Geometry: final body of the model. Coordinates: model frame, mm. Face numbers are marked on the shaded views. A direction names the side the tool comes from. Give positions to 0.01 mm unless a question says otherwise; leave off trailing zeros. Write each loop counter-clockwise with the first axis right and the second up, starting at its lowest first coordinate (ties: lowest second). Pieces come first, ordered by that corner, then holes.
Q1. Section A-A (y = 0). Return the cut outline in (x, z).
Q2. Mould query, pull axis Y, two halves, no side actions, for the marked faces 3, 4 and 5. Classes: +Y half, -Y half, draft (parallel to the pull), parting line (faces both ways), or undercut.
Q3. Section B-B (x = -35). Return the cut outline in (y, z).
Q4. Pin query (flat end, axial travel): pin 1 Ø5 at (y, z) = (-19, 38.5) entering from +X; pin 2 Ø1.4 at (x, y) = (0.5, -45.5) entering from -Z; pin 3 Ø6 at (x, y) = (-18.5, -7.5) entering from +Z; pin 4 Ø4 at (x, z) = (3, 8) entering from -Y. Return the tip coordinate at first contact, or that it passes through.
Q5. Section C-C (z = 40). Return the cut outline in (x, y).
Q6. Line query: line 1 (Y direction, x = 0, z = 55.5); line 2 (Z direction, x = 30, y = -27); line 3 (Y direction, x = 5, z = 57.5). Output: solid intervals per line, ascending.
Q7. Reachability of the marked faces 1 and 2 from +Z, -Z, +X, -X, +Y, -Y: full face, straight path, thin tool, end or side. Return the list, or none.
Q8. Section D-D (y = -37). Return the cut outline in (x, z).
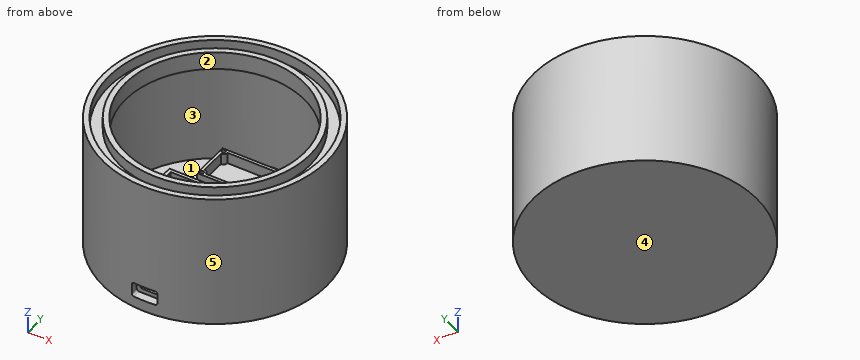
Autodesk Fusion 360 part; units mm, degrees
sketch "Boceto1" plane through (0, 0, 0) normal (0, 0, 1) x (1, 0, 0)
  circle A0 centre (0, 0) radius 50
  dimension "d4" = 100
extrude "Extruir1" add sketch "Boceto1" along normal blind 60
sketch "Boceto2" plane through (0, 0, 60) normal (0, 0, 1) x (-1, 0, 0)
  circle A0 centre (0, 0) radius 50
  circle A1 centre (0, 0) radius 47.5
  circle A2 centre (0, 0) radius 42.5
  circle A3 centre (0, 0) radius 40
  dimension "d7" = 95
  dimension "d8" = 85
  dimension "d9" = 80
extrude "Extruir2" cut sketch "Boceto2" against normal blind 5 contours A1 | A3
extrude "Extruir3" cut 1 faces at (-12.741, 3.9301, 55) along direction (0, 0, -1) blind 50
sketch "Boceto3" plane through (0, 0, 5) normal (0, 0, 1) x (-1, 0, 0)
  circle A0 centre (0, 0) radius 45
  dimension "d14" = 90
extrude "Extruir4" cut sketch "Boceto3" along normal blind 47
sketch "Boceto4" plane through (0, 0, 5) normal (0, 0, 1) x (-1, 0, 0)
  circle A0 centre (0, 0) radius 45
  line L0 (21.5929, -21.3537) -> (-21.6071, -21.3537)
  line L1 (-21.6071, -21.3537) -> (-21.6071, -39.3537)
  line L2 (-21.6071, -39.3537) -> (21.5929, -39.3537)
  line L3 (21.5929, -39.3537) -> (21.5929, -21.3537)
  line L4 (21.5929, -21.3537) -> (-21.6071, -39.3537) construction
  line L5 (-21.6071, -21.3537) -> (21.5929, -39.3537) construction
  line L6 (20.3129, -24.5337) -> (20.3129, -36.1737)
  line L7 (-20.3271, -36.1737) -> (-20.3271, -24.5337)
  line L8 (-20.3271, -22.7337) -> (20.3129, -37.9737) construction
  line L9 (20.3129, -22.7337) -> (-20.3271, -37.9737) construction
  circle A1 centre (20.3129, -37.9737) radius 0.9
  circle A2 centre (20.3129, -22.7337) radius 0.9
  circle A3 centre (-20.3271, -22.7337) radius 0.9
  circle A4 centre (-20.3271, -37.9737) radius 0.9
  arc A5 (20.3129, -36.1737) -> (18.5129, -37.9737) centre (20.3129, -37.9737) ccw
  arc A6 (18.5129, -22.7337) -> (20.3129, -24.5337) centre (20.3129, -22.7337) ccw
  arc A7 (-20.3271, -24.5337) -> (-18.5271, -22.7337) centre (-20.3271, -22.7337) ccw
  line L10 (-18.5271, -22.7337) -> (18.5129, -22.7337)
  arc A8 (-18.5271, -37.9737) -> (-20.3271, -36.1737) centre (-20.3271, -37.9737) ccw
  line L11 (18.5129, -37.9737) -> (-18.5271, -37.9737)
  point P0 (-0.0071, -30.3537)
  point P1 (-0.0071, -30.3537)
  dimension "d17" = 43.2
  dimension "d18" = 18
  dimension "d19" = 40.64
  dimension "d20" = 15.24
  dimension "d21" = 1.8
  dimension "d22" = 1.8
  dimension "d23" = 1.8
  dimension "d24" = 1.8
  dimension "d25" = 3.6
  dimension "d28" = 3.6
extrude "Extruir5" add sketch "Boceto4" along normal blind 5 contours L0 L1 L2 L3
thread "Rosca1"
sketch "Boceto5" plane through (0, 0, 5) normal (0, 0, 1) x (-1, 0, 0)
  circle A0 centre (0, 0) radius 45
  line L0 (21.5929, -39.3537) -> (-21.6071, -39.3537)
  line L1 (-21.6071, -39.3537) -> (-21.6071, -21.3537)
  line L2 (-21.6071, -21.3537) -> (21.5929, -21.3537)
  line L3 (21.5929, -21.3537) -> (21.5929, -39.3537)
  line L4 (32.8916, 28.8691) -> (9.8916, 28.8691)
  line L5 (9.8916, 28.8691) -> (9.8916, -19.6309)
  line L6 (9.8916, -19.6309) -> (32.8916, -19.6309)
  line L7 (32.8916, -19.6309) -> (32.8916, 28.8691)
  line L8 (32.8916, 28.8691) -> (9.8916, -19.6309) construction
  line L9 (9.8916, 28.8691) -> (32.8916, -19.6309) construction
  line L10 (32.8916, 28.8691) -> (32.8916, 20.6691)
  line L11 (30.8916, 20.6691) -> (29.8916, 20.6691)
  line L12 (9.8916, -19.6309) -> (9.8916, -12.1309)
  circle A1 centre (29.8916, 20.6691) radius 1
  line L13 (31.3916, 27.3691) -> (11.3916, 27.3691)
  line L14 (11.3916, -18.1309) -> (31.3916, -18.1309)
  line L15 (31.3916, 27.3691) -> (11.3916, -18.1309) construction
  line L16 (11.3916, 27.3691) -> (31.3916, -18.1309) construction
  line L17 (31.3916, 18.6691) -> (29.8916, 18.6691)
  line L18 (31.3916, 22.6691) -> (29.8916, 22.6691)
  arc A2 (29.951, 22.6682) -> (29.8916, 18.6691) centre (29.8916, 20.6691) ccw
  line L19 (31.3916, -18.1309) -> (31.3916, 18.6691)
  line L20 (31.3916, 22.6691) -> (31.3916, 27.3691)
  line L21 (11.3916, 27.3691) -> (11.3916, -9.9856)
  line L22 (11.3916, -14.1309) -> (11.3916, -18.1309)
  circle A3 centre (12.8916, -12.1309) radius 1
  line L23 (11.3916, -10.1309) -> (12.8916, -10.1309)
  line L24 (11.3916, -14.1309) -> (12.8916, -14.1309)
  line L25 (11.3916, -9.9856) -> (11.3916, -10.1309)
  arc A4 (12.8916, -14.1309) -> (12.8916, -10.1309) centre (12.8916, -12.1309) ccw
  point P0 (21.3916, 4.6191)
  point P1 (21.3916, 4.6191)
  dimension "d31" = 23
  dimension "d32" = 48.5
  dimension "d33" = 8.2
  dimension "d34" = 3
  dimension "d35" = 7.5
  dimension "d38" = 2
  dimension "d39" = 20
  dimension "d40" = 45.5
  dimension "d41" = 4
  dimension "d47" = 180
  dimension "d48" = 3
  dimension "d49" = 2
  dimension "d50" = 4
extrude "Extruir6" add sketch "Boceto5" along normal blind 3.5 contours L4 L5 L6 L7 L10 L12
ref_plane "PlanoDeObra1" through (0, -50, 0) normal (0, 1, 0) x (0, 0, 1)
sketch "Boceto6" plane through (0, -50, 0) normal (0, 1, 0) x (1, 0, 0)
  line L0 (0, 0) -> (0, -5)
  line L1 (0, -5) -> (5.75, -5)
  line L2 (0, -5) -> (-5.75, -5)
  line L3 (-5.75, -5) -> (-5.75, -11.5)
  line L4 (-5.75, -11.5) -> (5.75, -11.5)
  line L5 (5.75, -11.5) -> (5.75, -5)
  line L6 (3.1, -6.95) -> (-3.1, -6.95)
  line L7 (-4.2, -8.05) -> (-4.2, -8.45)
  line L8 (-3.1, -9.55) -> (3.1, -9.55)
  line L9 (4.2, -8.45) -> (4.2, -8.05)
  line L10 (4.2, -6.95) -> (-4.2, -9.55) construction
  line L11 (-4.2, -6.95) -> (4.2, -9.55) construction
  arc A0 (-4.2, -8.45) -> (-3.1, -9.55) centre (-3.1, -8.45) ccw
  arc A1 (-3.1, -6.95) -> (-4.2, -8.05) centre (-3.1, -8.05) ccw
  arc A2 (4.2, -8.05) -> (3.1, -6.95) centre (3.1, -8.05) ccw
  arc A3 (3.1, -9.55) -> (4.2, -8.45) centre (3.1, -8.45) ccw
  point P0 (0, -8.25)
  dimension "d56" = 5
  dimension "d57" = 5.75
  dimension "d58" = 5.75
  dimension "d59" = 6.5
  dimension "d60" = 11.5
  dimension "d61" = 8.4
  dimension "d62" = 2.6
  dimension "d65" = 1.1
  dimension "d66" = 1.1
  dimension "d67" = 1.1
  dimension "d68" = 1.1
extrude "Extruir7" cut sketch "Boceto6" along normal blind 3 contours L1 L2 L3 L4 L5 | L6 L7 L8 L9 A0 A1 A2 A3
sketch "Boceto7" plane through (0, -47, 0) normal (0, -1, 0) x (1, 0, 0)
  line L0 (-5.75, 5) -> (5.75, 5)
  line L1 (5.75, 5) -> (5.75, 11.5)
  line L2 (5.75, 11.5) -> (-5.75, 11.5)
  line L3 (-5.75, 11.5) -> (-5.75, 5)
  line L4 (3.1, 6.95) -> (-3.1, 6.95)
  line L5 (-4.2, 8.05) -> (-4.2, 8.45)
  line L6 (-3.1, 9.55) -> (3.1, 9.55)
  line L7 (4.2, 8.45) -> (4.2, 8.05)
  line L8 (4.2, 6.95) -> (-4.2, 9.55) construction
  line L9 (-4.2, 6.95) -> (4.2, 9.55) construction
  arc A0 (-3.1, 9.55) -> (-4.2, 8.45) centre (-3.1, 8.45) ccw
  arc A1 (-4.2, 8.05) -> (-3.1, 6.95) centre (-3.1, 8.05) ccw
  arc A2 (4.2, 8.45) -> (3.1, 9.55) centre (3.1, 8.45) ccw
  arc A3 (3.1, 6.95) -> (4.2, 8.05) centre (3.1, 8.05) ccw
  point P0 (0, 8.25)
  dimension "d71" = 8.4
  dimension "d72" = 2.6
  dimension "d73" = 1.1
  dimension "d74" = 1.1
  dimension "d75" = 1.1
extrude "Extruir8" cut sketch "Boceto7" against normal blind 2.3 contours L4 L5 L6 L7 A0 A1 A2 A3
fillet "Empalme1" radius 1 4 edges at (-5.75, -48.3341, 11.5) (-5.75, -48.3341, 5) (5.75, -48.3341, 5) (5.75, -48.3341, 11.5)
extrude "Extruir9" cut 1 faces at (1.0333, -47, 10.85) along direction (0, 1, 0) blind 0.826
sketch "Boceto8" plane through (0, 0, 5) normal (0, 0, 1) x (-1, 0, 0)
  line L0 (21.5929, -39.3537) -> (-21.6071, -39.3537)
  line L1 (-21.6071, -39.3537) -> (-21.6071, -21.3537)
  line L2 (-21.6071, -21.3537) -> (21.5929, -21.3537)
  line L3 (21.5929, -21.3537) -> (21.5929, -39.3537)
  circle A0 centre (0, 0) radius 45
  line L4 (32.8916, -19.6309) -> (9.8916, -19.6309)
  line L5 (9.8916, -19.6309) -> (9.8916, 28.8691)
  line L6 (9.8916, 28.8691) -> (32.8916, 28.8691)
  line L7 (32.8916, 28.8691) -> (32.8916, -19.6309)
  line L8 (0, 45) -> (-5.47, 45)
  line L9 (0, 45) -> (5.47, 45)
  line L10 (-5.47, 45) -> (-5.47, 39.05)
  line L11 (-5.47, 39.05) -> (5.47, 39.05)
  line L12 (5.47, 39.05) -> (5.47, 45)
  dimension "d83" = 5.47
  dimension "d84" = 5.47
  dimension "d85" = 5.95
  dimension "d86" = 10.94
extrude "Extruir10" add sketch "Boceto8" along normal blind 1 contours A0 L10 L11 L12 picked at (0, 41.0333)
equation "DiametroBase = 100 mm"
equation "AlturaBase = 60 mm"
equation "AlturaPantalla = 200 mm"
equation "d4 = DiametroBase"
equation "d5 = AlturaBase"
Computed:
1. outline: (-50, 0) - (50, 0) - (50, 60) - (47.5, 60) - (47.5, 55) - (42.5, 55) - (42.5, 60) - (40, 60) - (40, 52) - (45, 52) - (45, 5) - (-9.89, 5) - (-9.89, 8.5) - (-11.39, 8.5) - (-11.39, 5) - (-31.39, 5) - (-31.39, 8.5) - (-32.89, 8.5) - (-32.89, 5) - (-45, 5) - (-45, 52) - (-40, 52) - (-40, 60) - (-42.5, 60) - (-42.5, 55) - (-47.5, 55) - (-47.5, 60) - (-50, 60) - close
2. face 3: undercut
2. face 4: draft
2. face 5: parting line
3. outline: (-35.71, 0) - (35.71, 0) - (35.71, 60) - (32.11, 60) - (32.11, 55) - (24.11, 55) - (24.11, 60) - (19.36, 60) - (19.36, 52) - (28.28, 52) - (28.28, 5) - (-28.28, 5) - (-28.28, 52) - (-19.36, 52) - (-19.36, 60) - (-24.11, 60) - (-24.11, 55) - (-32.11, 55) - (-32.11, 60) - (-35.71, 60) - close
4. pin 1: stops at x = 47.2
4. pin 2: stops at z = 0
4. pin 3: stops at z = 5
4. pin 4: stops at y = -46.17
5. outline: circle Ø100 at (0, 0); hole circle Ø90 at (0, 0)
6. line 1: y = -50 to -47.5, -42.5 to -40, 40 to 42.5, 47.5 to 50
6. line 2: z = 0 to 5, 52 to 60
6. line 3: y = -49.75 to -47.24, -42.2 to -39.69, 39.69 to 42.2, 47.24 to 49.75
7. face 1: none
7. face 2: +Z
8. outline: (-33.63, 0) - (33.63, 0) - (33.63, 60) - (29.79, 60) - (29.79, 55) - (20.91, 55) - (20.91, 60) - (15.2, 60) - (15.2, 52) - (25.61, 52) - (25.61, 5) - (-25.61, 5) - (-25.61, 52) - (-15.2, 52) - (-15.2, 60) - (-20.91, 60) - (-20.91, 55) - (-29.79, 55) - (-29.79, 60) - (-33.63, 60) - close
